```python
from build123d import *

# Parameters (mm, degrees)
F0_R     = 1.7272
F0_R_2   = 2.15265
F0_R_3   = 3.96875
F0_R_4   = 11.1125
F1_DEPTH = 3.175
F3_DEPTH = 3.175
F4_COUNT = 6
F4_ANGLE = 300


with BuildPart() as f1:
    # F0 (on Top) → F1 (new body)
    with BuildSketch(Plane.XY):
        with BuildLine():
            Line((-303.6125627, 32.54375), (-346.1094200534, 21.5120031198))
            ThreePointArc((-346.1094200534, 21.5120031198), (-362.7501254, 0), (-346.1094200534, -21.5120031198))
            Line((-346.1094200534, -21.5120031198), (-303.6125627, -32.54375))
            Line((-303.6125627, -32.54375), (-297.2625627, -32.54375))
            Line((-297.2625627, -32.54375), (-297.2625627, -29.36875))
            Line((-297.2625627, -29.36875), (-43.2625627, -29.36875))
            Line((-43.2625627, -29.36875), (-43.2625627, -32.54375))
            Line((-43.2625627, -32.54375), (-36.9125627, -32.54375))
            Line((-36.9125627, -32.54375), (-6.2993370693, -24.5968716335))
            ThreePointArc((-6.2993370693, -24.5968716335), (25.3907018743, 0), (-6.2993370693, 24.5968716335))
            Line((-6.2993370693, 24.5968716335), (-36.9125627, 32.54375))
            Line((-36.9125627, 32.54375), (-43.2625627, 32.54375))
            Line((-43.2625627, 32.54375), (-43.2625627, 29.36875))
            Line((-43.2625627, 29.36875), (-297.2625627, 29.36875))
            Line((-297.2625627, 29.36875), (-297.2625627, 32.54375))
            Line((-297.2625627, 32.54375), (-303.6125627, 32.54375))
        make_face()
        with Locations((-282.9750627, -24.60625)):
            Circle(F0_R, mode=Mode.SUBTRACT)
        with Locations((-352.8729798, -12.3478544)):
            Circle(F0_R_2, mode=Mode.SUBTRACT)
        with Locations((-328.177271, -12.3478544)):
            Circle(F0_R_3, mode=Mode.SUBTRACT)
        with Locations((-57.5500627, -24.60625)):
            Circle(F0_R, mode=Mode.SUBTRACT)
        with Locations((-12.3478544, -12.3478544)):
            Circle(F0_R_2, mode=Mode.SUBTRACT)
        with Locations((12.3478544, -12.3478544)):
            Circle(F0_R_2, mode=Mode.SUBTRACT)
        with Locations((-340.5251254, 0)):
            Circle(F0_R_4, mode=Mode.SUBTRACT)
        with Locations((-289.7251254, 0)):
            Circle(F0_R, mode=Mode.SUBTRACT)
        with Locations((-352.8729798, 12.3478544)):
            Circle(F0_R_3, mode=Mode.SUBTRACT)
        with Locations((-328.177271, 12.3478544)):
            Circle(F0_R_2, mode=Mode.SUBTRACT)
        with Locations((-282.9750627, 24.60625)):
            Circle(F0_R, mode=Mode.SUBTRACT)
        with Locations((-50.8, 0)):
            Circle(F0_R, mode=Mode.SUBTRACT)
        Circle(F0_R_4, mode=Mode.SUBTRACT)
        with Locations((-12.3478544, 12.3478544)):
            Circle(F0_R_2, mode=Mode.SUBTRACT)
        with Locations((12.3478544, 12.3478544)):
            Circle(F0_R_2, mode=Mode.SUBTRACT)
        with Locations((-57.5500627, 24.60625)):
            Circle(F0_R, mode=Mode.SUBTRACT)
    extrude(amount=F1_DEPTH)

    # F2 (on face) → F3 (cut, through all)
    with BuildSketch(Plane(origin=(0, 0, 0), x_dir=(1, 0, 0), z_dir=(0, 0, -1))):
        with BuildLine():
            ThreePointArc((-348.3828495059, -7.8577241059), (-350.1488326996, -5.55625), (-351.2589761446, -2.8761266387))
            Line((-351.2589761446, -2.8761266387), (-352.0256797693, -3.0815642558))
            ThreePointArc((-352.0256797693, -3.0815642558), (-350.8362403638, -5.953125), (-348.9441155135, -8.4189901135))
            Line((-348.9441155135, -8.4189901135), (-348.3828495059, -7.8577241059))
        make_face()
    f3 = extrude(amount=-F3_DEPTH, mode=Mode.SUBTRACT)

    # F4: F3 ×6 about axis
    f4_axis = Axis((-340.5251254, 0, 0), (0, 0, -1))
    for i in range(1, F4_COUNT):
        add(f3.rotate(f4_axis, i * F4_ANGLE / (F4_COUNT - 1)), mode=Mode.SUBTRACT)


solid = f1.part
```
Can you work these out from the model? Positions are in its coordinate system, mm. Round coordinates to 2 decimals unless told otherwise and drop trailing zeros. Loops run counter-clockwise (first coordinate to the right, second up) from the corner with the lowest first, then second, coordinate; pieces in that order, holes last.
Item 1: Please list where these lines run through material, in increasing order: L1, parallel to Y at x = -341, z = 1; L2, parallel to X at y = 4, z = 0.75; L3, parallel to X at y = 9.5, z = 2.55.
Item 2: Will these pins go through, and if not, where does the flat tip stop? pin 1 Ø1 at (x, z) = (-182.5, 2) entering from +Y; pin 2 Ø6.5 at (x, y) = (-352.87, 12.35) entering from +Z; pin 3 Ø1 at (x, z) = (-202.5, 2.5) entering from -Y.
Item 3: Suppose I cut it at B-B, the plane x = -116.5. Write out the boundary of the cut face in (y, z) (3 decimals).
Item 4: Suppose I cut it at D-D, the plane x = -320.5. Write out the boundary of the cut face in (y, z) (3 decimals).
Item 5: Suppose I cut it at C-C, the plane z = 2.5. State how many separate pieces and enclosed holes the cut face has, then the cut area to 3 significant figures.
Item 6: Suppose I cut it at A-A, the plane x = 0. Write out the boundary of the cut face in (y, z) (1 decimal), then the cut area to 3 significant figures.
Item 7: If we mould it in two halves opening along Y, with no side actions, what happens to faces 1 (the flat face through (-325.16, -26.95, 1.57)), 2 (the cylindrical face through (-362.746, 0.41, 1.565)), 3 (the cylindrical face through (-332.142, -12.173, 1.565))? For each: +Y half, -Y half, draft (parallel to the pull), parting line (faces both ways), or undercut.
Reported:
1. L1: y = -22.84 to -11.9, 11.9 to 22.84
1. L2: x = -362.39 to -351.74, -329.31 to -10.37, 10.37 to 25.07
1. L3: x = -360.62 to -355.64, -350.11 to -346.29, -334.76 to -5.77, 5.77 to 23.55
2. pin 1: stops at y = 29.37
2. pin 2: passes through
2. pin 3: stops at y = -29.37
3. outline: (-29.369, 0) - (29.369, 0) - (29.369, 3.175) - (-29.369, 3.175) - close
4. outline: (-28.16, 0) - (28.16, 0) - (28.16, 3.175) - (-28.16, 3.175) - close
5. separate pieces: 1
5. enclosed holes: 16
5. area: 20,600 mm2
6. outline: (-25.4, 0) - (-11.1, 0) - (-11.1, 3.2) - (-25.4, 3.2) - close; (11.1, 0) - (25.4, 0) - (25.4, 3.2) - (11.1, 3.2) - close
6. area: 90.7 mm2
7. face 1: -Y half
7. face 2: parting line
7. face 3: undercut
